```python
from build123d import *

# Parameters (mm, degrees)
SKETCH1_W           = 53.89
SKETCH1_H           = 40
BOSS_EXTRUDE1_DEPTH = 3
SKETCH2_R           = 2.25
SKETCH2_W           = 3
SKETCH2_H           = 5
CUT_EXTRUDE1_DEPTH  = 3


with BuildPart() as part:
    # Sketch1 → Boss-Extrude1 (new body)
    with BuildSketch(Plane.XY):
        Rectangle(SKETCH1_W, SKETCH1_H)
    extrude(amount=BOSS_EXTRUDE1_DEPTH)

    # Sketch2 → Cut-Extrude1 (cut)
    with BuildSketch(Plane.XY.offset(3)):
        with Locations((-10.495, 11.5)):
            Circle(SKETCH2_R)
        with Locations((-25.445, 17.5)):
            Rectangle(SKETCH2_W, SKETCH2_H)
        with Locations((-25.445, 7.5)):
            Rectangle(SKETCH2_W, SKETCH2_H)
        with Locations((25.445, 17.5)):
            Rectangle(SKETCH2_W, SKETCH2_H)
        with Locations((25.445, 7.5)):
            Rectangle(SKETCH2_W, SKETCH2_H)
        with Locations((25.445, -2.5)):
            Rectangle(SKETCH2_W, SKETCH2_H)
        with Locations((-25.445, -2.5)):
            Rectangle(SKETCH2_W, SKETCH2_H)
    extrude(amount=-CUT_EXTRUDE1_DEPTH, mode=Mode.SUBTRACT)


solid = part.part
```
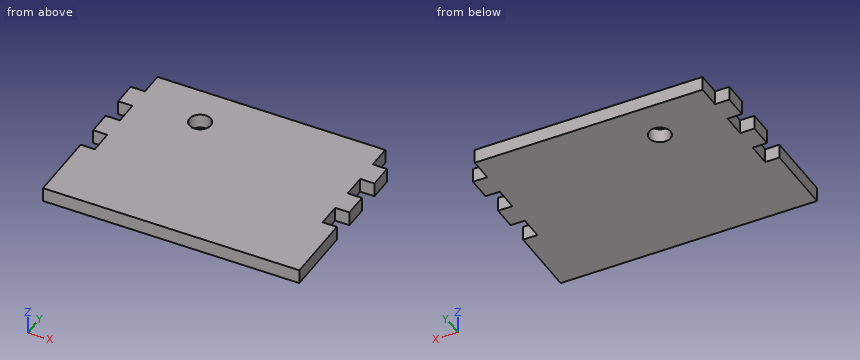
For this review, take the finished solid that the model builds, in its own axes (mm). Round coordinates to 2 decimals unless told otherwise and drop trailing zeros. Order: outer loops, then holes, each group sorted by start corner. A loop starts at its lowest first (then second) coordinate and runs counter-clockwise, first axis right, second up.
Q1. Insertion check: P1, Ø1.5, axis at y = 18, z = 1, coming from the +X side (3 decimals); P2, Ø1.5, axis at x = -26, z = 1, coming from the +Y side; P3, Ø0.9, axis at y = -3, z = 2, coming from the -X side (3 decimals). Each pin has a flat end and moves straight along its axis. Give the tip position at first contact, or say it passes through.
Findings below:
P1: stops at x = 23.945
P2: stops at y = 15
P3: stops at x = -23.945
Q2. We need section C-C, the plane y = -1.5. Give the boundary of the cut face in (x, z) (3 decimals), plus the area to 3 significant figures.
Findings below:
outline: (-23.945, 0) - (23.945, 0) - (23.945, 3) - (-23.945, 3) - close
area: 144 mm2
Q3. Wall thickness on line 1 (Y direction, x = -9, z = 2.85); line 2 (X direction, y = 9, z = 0.9) (3 decimals): over which ranges is each line inside the solid? List them lowest first.
Findings below:
line 1: y = -20 to 9.82, 13.18 to 20
line 2: x = -23.945 to 23.945
Q4. We need section B-B, the plane z = 1.4. Give the boundary of the cut face in (x, y) (3 decimals), plus the area to 3 significant figures.
Findings below:
outline: (-26.945, -20) - (26.945, -20) - (26.945, -5) - (23.945, -5) - (23.945, 0) - (26.945, 0) - (26.945, 5) - (23.945, 5) - (23.945, 10) - (26.945, 10) - (26.945, 15) - (23.945, 15) - (23.945, 20) - (-23.945, 20) - (-23.945, 15) - (-26.945, 15) - (-26.945, 10) - (-23.945, 10) - (-23.945, 5) - (-26.945, 5) - (-26.945, 0) - (-23.945, 0) - (-23.945, -5) - (-26.945, -5) - close; hole circle Ø4.5 at (-10.495, 11.5)
area: 2,050 mm2
Q5. We need section A-A, the plane y = 11.5. Give the boundary of the cut face in (x, z) (3 decimals).
Findings below:
outline: (-26.945, 0) - (-12.745, 0) - (-12.745, 3) - (-26.945, 3) - close; (-8.245, 0) - (26.945, 0) - (26.945, 3) - (-8.245, 3) - close
